Source: CAD feature listing. Evaluate the final solid. Frame: model axes, mm. Give positions to 0.01 mm unless a question says otherwise; leave off trailing zeros. Order: outer loops, then holes, each group sorted by start corner. A loop starts at its lowest first (then second) coordinate and runs counter-clockwise, first axis right, second up.
Autodesk Inventor part; units mm, degrees
ref_plane "YZ Plane" through (0, 0, 0) normal (1, 0, 0) x (0, 1, 0)
ref_plane "XZ Plane" through (0, 0, 0) normal (0, 1, 0) x (-1, 0, 0)
ref_plane "XY Plane" through (0, 0, 0) normal (0, 0, 1) x (1, 0, 0)
sketch "Sketch1" plane through (0, 0, 0) normal (0, 1, 0) x (-1, 0, 0)
  circle A0 centre (0, 0) radius 34
  circle A1 centre (9.5, 0) radius 1.6
  circle A2 centre (4.75, 8.2272) radius 1.6
  circle A3 centre (-4.75, 8.2272) radius 1.6
  circle A4 centre (-9.5, 0) radius 1.6
  circle A5 centre (-4.75, -8.2272) radius 1.6
  circle A6 centre (4.75, -8.2272) radius 1.6
  circle A7 centre (30, 0) radius 1.2
  circle A8 centre (21.2132, 21.2132) radius 1.2
  circle A9 centre (0, 30) radius 1.2
  circle A10 centre (-21.2132, 21.2132) radius 1.2
  circle A11 centre (-30, 0) radius 1.2
  circle A12 centre (-21.2132, -21.2132) radius 1.2
  circle A13 centre (0, -30) radius 1.2
  circle A14 centre (21.2132, -21.2132) radius 1.2
  dimension "d0" = 68
  dimension "d1" = 3.2
  dimension "d2" = 9.5
  dimension "d3" = 0
  dimension "d6" = 360
  dimension "d10" = 2.4
  dimension "d11" = 0
  dimension "d12" = 30
  dimension "d15" = 360
extrude "Extrusion3" add sketch "Sketch1" along normal blind 5
sketch "Sketch5" plane through (0, 0, 0) normal (0, -1, 0) x (1, 0, 0)
  circle A0 centre (0, 0) radius 34
  circle A1 centre (21.2132, 21.2132) radius 1.2
  circle A2 centre (30, 0) radius 1.2
  circle A3 centre (21.2132, -21.2132) radius 1.2
  circle A4 centre (0, -30) radius 1.2
  circle A5 centre (-21.2132, -21.2132) radius 1.2
  circle A6 centre (-30, 0) radius 1.2
  circle A7 centre (-21.2132, 21.2132) radius 1.2
  circle A8 centre (0, 30) radius 1.2
  circle A9 centre (0, 0) radius 27
  circle A10 centre (21.2132, 21.2132) radius 1.2
  circle A11 centre (30, 0) radius 1.2
  circle A12 centre (21.2132, -21.2132) radius 1.2
  circle A13 centre (0, -30) radius 1.2
  circle A14 centre (-21.2132, -21.2132) radius 1.2
  circle A15 centre (-30, 0) radius 1.2
  circle A16 centre (-21.2132, 21.2132) radius 1.2
  circle A17 centre (0, 30) radius 1.2
  circle A18 centre (0, 30) radius 1.225
  circle A19 centre (0, 0) radius 34
  dimension "d21" = 54
extrude "Extrusion4" add sketch "Sketch5" along normal blind 26.68 contours A0 | A18
sketch "Sketch6" plane through (0, 5, 0) normal (0, 1, 0) x (1, 0, 0)
  circle A0 centre (0, 0) radius 34
extrude "Extrusion5" cut sketch "Sketch6" against normal blind 5
properties part number "sprocketsHolder" material "ABS Plastic"
1) Section query C-C, the plane z = -30. Return the cut outline in (x, y), and give its area (3 significant figures).
Report:
outline: (-16, -26.68) - (-1.2, -26.68) - (-1.2, 0) - (-16, 0) - close; (1.2, -26.68) - (16, -26.68) - (16, 0) - (1.2, 0) - close
area: 790 mm2
2) Draft query along Z for faces 1 (the cylindrical face through (-0.16, -13.15, -31.19)), 2 (the flat face through (15, -26.68, -23)), 3 (the cylindrical face through (18.28, -13.15, -28.67)). Return one class per face: +Z half, -Z half, draft (parallel to the pull), parting line (faces both ways), or undercut.
Report:
face 1: undercut
face 2: draft
face 3: parting line
3) Section query B-B, the plane x = -30. Return the cut outline in (y, z), and give its area (3 significant figures).
Report:
outline: (-26.68, -16) - (0, -16) - (0, -1.2) - (-26.68, -1.2) - close; (-26.68, 1.2) - (0, 1.2) - (0, 16) - (-26.68, 16) - close
area: 790 mm2
4) Section query D-D, the plane x = 0. Return the cut outline in (y, z).
Report:
outline: (-26.68, -34) - (0, -34) - (0, -31.2) - (-26.68, -31.2) - close; (-26.68, -28.8) - (0, -28.8) - (0, -27) - (-26.68, -27) - close; (-26.68, 27) - (0, 27) - (0, 28.8) - (-26.68, 28.8) - close; (-26.68, 31.2) - (0, 31.2) - (0, 34) - (-26.68, 34) - close
5) Section query A-A, the plane z = 0. Return the cut outline in (x, y).
Report:
outline: (-34, -26.68) - (-31.2, -26.68) - (-31.2, 0) - (-34, 0) - close; (-28.8, -26.68) - (-27, -26.68) - (-27, 0) - (-28.8, 0) - close; (27, -26.68) - (28.8, -26.68) - (28.8, 0) - (27, 0) - close; (31.2, -26.68) - (34, -26.68) - (34, 0) - (31.2, 0) - close
6) Material intervals for L1, parallel to Z at x = 0, y = -6.75; L2, parallel to X at y = -12.25, z = -24; L3, parallel to X at y = -5.75, z = 22, sorted ascending.
Report:
L1: z = -34 to -31.2, -28.8 to -27, 27 to 28.8, 31.2 to 34
L2: x = -24.08 to -12.37, 12.37 to 24.08
L3: x = -25.92 to -22.12, -20.31 to -15.65, 15.65 to 20.31, 22.12 to 25.92
7) Pin query (flat end, axial travel): pin 1 (5 mm diameter, centred on x = 6, y = -13, fed in from -Z); pin 2 (12 mm diameter, centred on y = -19, z = 21.5, fed in from +X); pin 3 (2 mm diameter, centred on x = 21.21, z = 21.21, fed in from -Y); pin 4 (2 mm diameter, centred on y = -14, z = -2.5, fed in from -X). Return the tip coordinate at first contact, or that it passes through.
Report:
pin 1: stops at z = -33.82
pin 2: stops at x = 30.26
pin 3: passes through
pin 4: stops at x = -33.97
